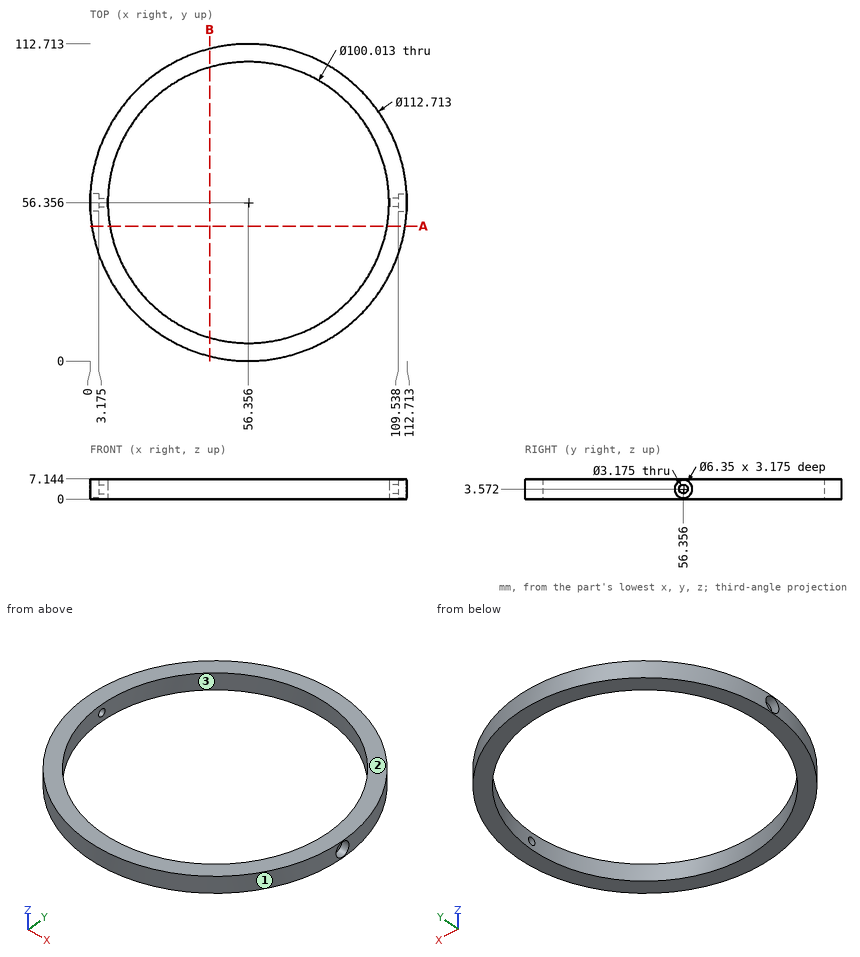
Could you check a few things on this drawing? It's one solid part, dimensions in mm from its lowest x, y, z. Round coordinates to 2 decimals unless told otherwise and drop trailing zeros. Loops run counter-clockwise (first coordinate to the right, second up) from the corner with the lowest first, then second, coordinate; pieces in that order, holes last.
Q1. Thinking about a two-plate mould opening in Y: for the marked faces 1, 2 and 3, which applies, pulls with the +Y half, pulls with the -Y half, needs draft (parallel to the pull), parting line crosses it, or undercut?
Q2. I want a section at B-B (x = 42.5). Write out the boundary of the cut face in (y, z) (1 decimal).
Q3. I want a section at A-A (y = 48). Write out the boundary of the cut face in (x, z).
Q4. Please list where these lines run through material, in increasing order: L1, parallel to Y at x = 58, z = 2.25 (1 decimal); L2, parallel to Y at x = 75, z = 4.75 (1 decimal); L3, parallel to X at y = 37.5, z = 6 (1 decimal).
Q5. For P1, Ø3, axis at x = 15, z = 5.5, coming from the -Y side; P2, Ø1, axis at y = 37, z = 6, coming from the +X side (1 decimal); P3, Ø3, axis at y = 33, z = 3, coming from the +X side, each with a flat end and sliding along its axis, tell me the tip position at first contact or that it passes through.
Answer below:
1. face 1: parting line crosses it
1. face 2: needs draft
1. face 3: undercut
2. outline: (1.7, 0) - (8.3, 0) - (8.3, 7.1) - (1.7, 7.1) - close; (104.4, 0) - (111, 0) - (111, 7.1) - (104.4, 7.1) - close
3. outline: (0.62, 0) - (7.05, 0) - (7.05, 7.14) - (0.62, 7.14) - close; (105.66, 0) - (112.09, 0) - (112.09, 7.14) - (105.66, 7.14) - close
4. L1: y = 0 to 6.4, 106.3 to 112.7
4. L2: y = 3.2 to 10, 102.8 to 109.5
4. L3: x = 3.2 to 10, 102.7 to 109.5
5. P1: stops at y = 16.51
5. P2: stops at x = 109.5
5. P3: stops at x = 108.3
